The model under review builds one solid part; all positions refer to its coordinate system, in mm. Round coordinates to 2 decimals unless told otherwise and drop trailing zeros. Order: outer loops, then holes, each group sorted by start corner. A loop starts at its lowest first (then second) coordinate and runs counter-clockwise, first axis right, second up.
1) Consider section B-B (x = 4). Give the boundary of the cut face in (y, z).
2) Clearance check with a flat-ended pin moving along its axis: P1, Ø0.9, axis at x = 0.5, y = 1, coming from the -Z side (3 decimals). State where the tip first meets the part, or that it passes through.
3) Consider section A-A (z = -6.25). Give the boundary of the cut face in (x, y).
4) Consider section D-D (x = -10.5). Give the boundary of the cut face in (y, z), then the cut area to 3 significant figures.
5) Consider section C-C (z = 4). Give the boundary of the cut face in (x, y), then the cut area to 3 significant figures.
6) To check wall thickness, follow L1, parallel to X at y = 1.4, z = 4.75; L2, parallel to Z at x = 3.75, y = 1.1; L3, parallel to Z at x = -6, y = 1.45. State the ranges of each line that lie inside material, in increasing order.
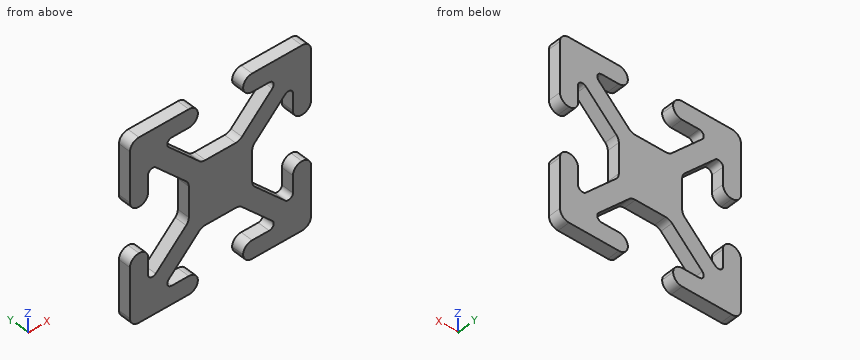
Autodesk Inventor part; units mm, degrees
ref_plane "YZ Plane" through (0, 0, 0) normal (1, 0, 0) x (0, 1, 0)
ref_plane "XZ Plane" through (0, 0, 0) normal (0, 1, 0) x (-1, 0, 0)
ref_plane "XY Plane" through (0, 0, 0) normal (0, 0, 1) x (1, 0, 0)
sketch "Sketch1" plane through (0, 0, 0) normal (0, 1, 0) x (-1, 0, 0)
  line L0 (12.7, 12.7) -> (-12.7, 12.7)
  line L1 (-12.7, 12.7) -> (-12.7, -12.7)
  line L2 (-12.7, -12.7) -> (12.7, -12.7)
  line L3 (12.7, -12.7) -> (12.7, 12.7)
  line L4 (12.7, 12.7) -> (-12.7, -12.7) construction
  line L5 (-12.7, 12.7) -> (12.7, -12.7) construction
  line L6 (10.16, 10.16) -> (-10.16, 10.16)
  line L7 (-10.16, 10.16) -> (-10.16, -10.16)
  line L8 (-10.16, -10.16) -> (10.16, -10.16)
  line L9 (10.16, -10.16) -> (10.16, 10.16)
  line L10 (10.16, 10.16) -> (-10.16, -10.16) construction
  line L11 (-10.16, 10.16) -> (10.16, -10.16) construction
  line L12 (-4.445, 4.445) -> (4.445, 4.445)
  line L13 (4.445, 4.445) -> (4.445, -4.445)
  line L14 (4.445, -4.445) -> (-4.445, -4.445)
  line L15 (-4.445, -4.445) -> (-4.445, 4.445)
  line L16 (-4.445, 4.445) -> (4.445, -4.445) construction
  line L17 (4.445, 4.445) -> (-4.445, -4.445) construction
  line L18 (0, 12.7) -> (-3.175, 12.7)
  line L19 (-3.175, 12.7) -> (3.175, 12.7)
  line L20 (3.175, 12.7) -> (3.175, -12.7)
  line L21 (3.175, -12.7) -> (-3.175, -12.7)
  line L22 (-3.175, -12.7) -> (-3.175, 12.7)
  line L23 (12.7, 0) -> (12.7, 3.175)
  line L24 (12.7, 3.175) -> (-12.7, 3.175)
  line L25 (-12.7, 3.175) -> (-12.7, -3.175)
  line L26 (-12.7, -3.175) -> (12.7, -3.175)
  line L27 (12.7, -3.175) -> (12.7, 3.175)
  line L28 (-13.598, -11.802) -> (11.802, 13.598)
  line L29 (11.802, 13.598) -> (13.598, 11.802)
  line L30 (13.598, 11.802) -> (-11.802, -13.598)
  line L31 (-11.802, -13.598) -> (-13.598, -11.802)
  line L32 (-13.598, -11.802) -> (13.598, 11.802) construction
  line L33 (11.802, 13.598) -> (-11.802, -13.598) construction
  line L34 (-13.598, 11.802) -> (11.802, -13.598)
  line L35 (11.802, -13.598) -> (13.598, -11.802)
  line L36 (13.598, -11.802) -> (-11.802, 13.598)
  line L37 (-11.802, 13.598) -> (-13.598, 11.802)
  line L38 (-13.598, 11.802) -> (13.598, -11.802) construction
  line L39 (11.802, -13.598) -> (-11.802, 13.598) construction
  point P0 (0, 0)
  point P1 (8.3639, 10.16)
  point P2 (2.6489, 4.445)
  point P3 (-2.6489, 4.445)
  point P4 (-8.3639, 10.16)
  point P5 (-10.16, 3.175)
  point P6 (-10.16, 8.3639)
  point P7 (-4.445, 2.6489)
  point P8 (-4.445, -2.6489)
  point P9 (-10.16, -8.3639)
  point P10 (-10.16, -3.175)
  point P11 (-3.175, -10.16)
  point P12 (-8.3639, -10.16)
  point P13 (-2.6489, -4.445)
  point P14 (2.6489, -4.445)
  point P15 (8.3639, -10.16)
  point P16 (3.175, -10.16)
  point P17 (10.16, -3.175)
  point P18 (10.16, -8.3639)
  point P19 (4.445, -2.6489)
  point P20 (4.445, 2.6489)
  point P21 (10.16, 8.3639)
  point P22 (10.16, 3.175)
  point P23 (-3.175, 10.16)
  point P24 (3.175, 10.16)
  dimension "d0" = 25.4
  dimension "d1" = 25.4
  dimension "d2" = 20.32
  dimension "d3" = 20.32
  dimension "d4" = 8.89
  dimension "d5" = 8.89
  dimension "d6" = 3.175
  dimension "d7" = 6.35
  dimension "d8" = 3.175
  dimension "d9" = 6.35
  dimension "d10" = 2.54
  dimension "d11" = 2.54
extrude "Extrusion1" add sketch "Sketch1" along normal blind 1.7526 contours L0 L28 L6 L20 | L0 L3 L30 L9 L6 L28 | L22 L6 L36 L0 | L6 L9 L30 L24 L13 L12 L20 L28 | L20 L12 L28 | L36 L6 L7 L34 L1 L0 | L3 L24 L9 L30 | L36 L22 L12 L15 L24 L34 L7 L6 | L36 L12 L22 | L20 L24 L28 L12 | L12 L13 L24 L20 | L28 L24 L36 L12 | L22 L24 L15 L12 | L12 L36 L24 L22 | L24 L13 L30 L20 | L20 L30 L36 L28 L24 | L28 L36 L24 | L34 L7 L24 L1 | L30 L13 L24 | L24 L36 L28 L34 L22 | L22 L34 L15 L24 | L30 L13 L36 L20 | L20 L36 L30 | L36 L30 L34 L28 | L3 L36 L9 L26 | L24 L15 L34 | L34 L28 L22 | L22 L28 L15 L34 | L36 L13 L26 L20 | L20 L26 L34 L30 L36 | L34 L30 L26 L22 L28 | L26 L7 L28 L1 | L3 L2 L34 L8 L9 L36 | L9 L8 L34 L20 L14 L13 L26 L36 | L26 L13 L36 | L22 L26 L15 L28 | L26 L13 L14 L20 | L20 L14 L34 L26 | L34 L26 L30 | L28 L7 L8 L30 L2 L1 | L28 L26 L15 L14 L22 L30 L8 L7 | L28 L15 L26 | L26 L30 L14 L22 | L22 L14 L15 L26 | L20 L34 L14 | L34 L14 L30 L26 | L2 L20 L8 L34 | L14 L30 L22 | L30 L8 L22 L2
fillet "Fillet1" radius 1.27 28 edges at (-12.7, 0.8763, -12.7) (12.7, 0.8763, -12.7) (3.175, 0.8763, -12.7) (3.175, 0.8763, -10.16) (-3.175, 0.8763, -12.7) (-12.7, 0.8763, -3.175) (-12.7, 0.8763, 3.175) (-10.16, 0.8763, 3.175) (-12.7, 0.8763, 12.7) (-3.175, 0.8763, 10.16) (3.175, 0.8763, 12.7) (3.175, 0.8763, 10.16) (10.16, 0.8763, 3.175) (12.7, 0.8763, 3.175) (10.16, 0.8763, -3.175) (12.7, 0.8763, -3.175) (12.7, 0.8763, 12.7) (-3.175, 0.8763, -10.16) (-10.16, 0.8763, -3.175) (-4.445, 0.8763, 2.6489) (-4.445, 0.8763, -2.6489) (2.6489, 0.8763, -4.445) (-2.6489, 0.8763, -4.445) (4.445, 0.8763, 2.6489) (4.445, 0.8763, -2.6489) (-2.6489, 0.8763, 4.445) (2.6489, 0.8763, 4.445) (-3.175, 0.8763, 12.7)
fillet "Fillet2" radius 0.635 8 edges at (8.3639, 0.8763, 10.16) (10.16, 0.8763, 8.3639) (-8.3639, 0.8763, 10.16) (-10.16, 0.8763, 8.3639) (-10.16, 0.8763, -8.3639) (-8.3639, 0.8763, -10.16) (8.3639, 0.8763, -10.16) (10.16, 0.8763, -8.3639)
properties part number "T_slot_1in_base" material "Aluminum 6061"
Answer below:
1. outline: (0, -12.62) - (1.75, -12.62) - (1.75, -10.24) - (0, -10.24) - close; (0, -5.8) - (1.75, -5.8) - (1.75, 5.8) - (0, 5.8) - close; (0, 10.24) - (1.75, 10.24) - (1.75, 12.62) - (0, 12.62) - close
2. P1: stops at z = -4.445
3. outline: (-12.7, 0) - (-10.16, 0) - (-10.16, 1.75) - (-12.7, 1.75) - close; (-8.05, 0) - (-4.45, 0) - (-4.45, 1.75) - (-8.05, 1.75) - close; (4.45, 0) - (8.05, 0) - (8.05, 1.75) - (4.45, 1.75) - close; (10.16, 0) - (12.7, 0) - (12.7, 1.75) - (10.16, 1.75) - close
4. outline: (0, -12.7) - (1.75, -12.7) - (1.75, -3.58) - (0, -3.58) - close; (0, 3.58) - (1.75, 3.58) - (1.75, 12.7) - (0, 12.7) - close
4. area: 32.0 mm2
5. outline: (-12.62, 0) - (-10.24, 0) - (-10.24, 1.75) - (-12.62, 1.75) - close; (-5.8, 0) - (5.8, 0) - (5.8, 1.75) - (-5.8, 1.75) - close; (10.24, 0) - (12.62, 0) - (12.62, 1.75) - (10.24, 1.75) - close
5. area: 28.7 mm2
6. L1: x = -12.7 to -10.16, -6.55 to -2.95, 2.95 to 6.55, 10.16 to 12.7
6. L2: z = -12.49 to -10.37, -5.55 to 5.55, 10.37 to 12.49
6. L3: z = -12.7 to -10.16, -7.8 to -4.2, 4.2 to 7.8, 10.16 to 12.7
